Design review of the part built by this model. Coordinates are the model's own, in mm. Face numbers are marked on the shaded views. A direction names the side the tool comes from. Give positions to 0.01 mm unless a question says otherwise; leave off trailing zeros. Loops run counter-clockwise (first coordinate to the right, second up) from the corner with the lowest first, then second, coordinate; pieces in that order, holes last. Notation, with made-up numbers: (63, 8.25) -> (81, 8.25) arc R16 ccw to (81, 21.25) -> close; hole circle Ø5 at (82, 4). An arc over 180 degrees is marked (long way). Answer in a Markdown table with one row per item. Add a question column.
(1) Consider section B-B on z = -11. Write out the cut boundary in (x, y), then the cut area to 3 significant figures.
(2) For line 1 (Z direction, x = 10.5, y = -5.75); line 2 (X direction, y = -12, z = -13.5); line 3 (X direction, y = -15.75, z = -9.75), list the stretches that pass through material, from the lowest coordinate up.
(3) Draft analysis for pull direction X (two halves, no side actions). For the marked faces 1, 2 and 3, state which applies: +X half, -X half, draft (parallel to the pull), parting line (faces both ways), or undercut.
(4) For pin 1 (2 mm diameter, centred on x = 17, y = -15, fed in from -Z); pin 2 (5 mm diameter, centred on x = 33.5, y = -13.5, fed in from -Z); pin 3 (3 mm diameter, centred on y = -20.5, z = -11, fed in from -X), all flat-tipped, find the tip position at first contact; note any pin that passes through.
(5) Consider section C-C on z = -8. Write out the cut boundary in (x, y).
(6) For the marked faces 4 and 5, list the 3-axis set-ups (+Z, -Z, +X, -X, +Y, -Y) from which the entire face can be reached by the end or side of a thin tool; tool diameter is ignored.
(7) Consider section D-D on z = -13.5. Write out the cut boundary in (x, y), then the cut area to 3 significant figures.
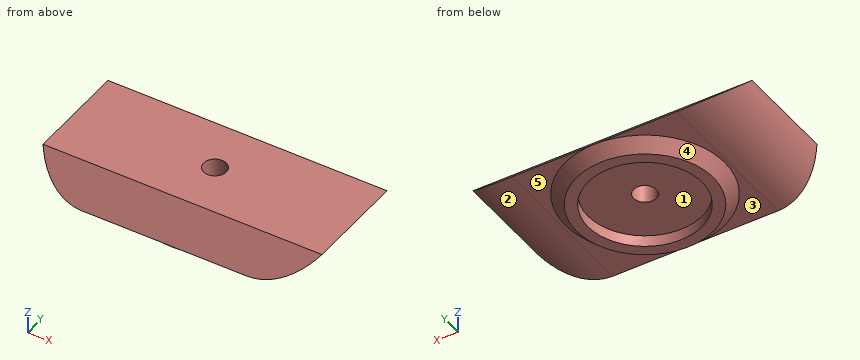
from build123d import *

# Parameters (mm, degrees)
PAD_DEPTH       = 28
SKETCH001_R     = 14
SKETCH001_R_2   = 10
PAD001_DEPTH    = 2
CHAMFER_SIZE    = 1.9999
CHAMFER001_SIZE = 4.9999
SKETCH002_R     = 2
POCKET_DEPTH    = 10


with BuildPart() as part:
    # Sketch → Pad (new body)
    with BuildSketch(Plane.XZ):
        with BuildLine():
            ThreePointArc((-10, -7.5), (-5.59017, -11.18034), (0, -12.5))
            Line((0, -12.5), (29.04, -12.5))
            ThreePointArc((29.04, -12.5), (34.63017, -11.18034), (39.04, -7.5))
            Line((-10, -7.5), (39.04, -7.5))
        make_face()
    extrude(amount=PAD_DEPTH)

    # Sketch001 (on Face2 of Pad) → Pad001 (join)
    with BuildSketch(Plane(origin=(0, 0, -12.5), x_dir=(1, 0, 0), z_dir=(0, 0, -1))):
        with Locations((14.52, 14)):
            Circle(SKETCH001_R)
        with Locations((14.52, 14)):
            Circle(SKETCH001_R_2, mode=Mode.SUBTRACT)
    extrude(amount=PAD001_DEPTH)

    # Chamfer
    chamfer_edges = [part.edges().sort_by_distance(p)[0] for p in [
        (0.52, -14, -14.5),
    ]]
    chamfer(chamfer_edges, length=CHAMFER_SIZE)

    # Chamfer001
    chamfer001_edges = [part.edges().sort_by_distance(p)[0] for p in [
        (14.52, 0, -7.5),
        (14.52, -28, -7.5),
    ]]
    chamfer(chamfer001_edges, length=CHAMFER001_SIZE)

    # Sketch002 (on Face14 of Chamfer001) → Pocket (cut)
    with BuildSketch(Plane(origin=(0, 0, -12.5), x_dir=(1, 0, 0), z_dir=(0, 0, -1))):
        with Locations((14.52, 14)):
            Circle(SKETCH002_R)
    extrude(amount=-POCKET_DEPTH, mode=Mode.SUBTRACT)


solid = part.part
Values follow:
| question | item | result |
|---|---|---|
| 1 | outline | (-5.94, -26.5) -> (34.98, -26.5) -> (34.98, -1.5) -> (-5.94, -1.5) -> close; hole circle Ø4 at (14.52, -14) |
| 1 | area | 1,010 mm2 |
| 2 | line 1 | -12.5 to -7.5 |
| 2 | line 2 | 1.67 to 4.72, 24.32 to 27.37 |
| 2 | line 3 | -7.82 to 13.55, 15.49 to 36.86 |
| 3 | face 1 | undercut |
| 3 | face 2 | +X half |
| 3 | face 3 | draft |
| 4 | pin 1 | z = -12.5 |
| 4 | pin 2 | z = -12.35 |
| 4 | pin 3 | x = -8.12 |
| 5 | outline | (-9.6, -23.5) -> (38.64, -23.5) -> (38.64, -4.5) -> (-9.6, -4.5) -> close; hole circle Ø4 at (14.52, -14) |
| 6 | face 4 | -Z |
| 6 | face 5 | -Z, +X |
| 7 | outline | circle Ø26 at (14.52, -14); hole circle Ø20 at (14.52, -14) |
| 7 | area | 217 mm2 |
